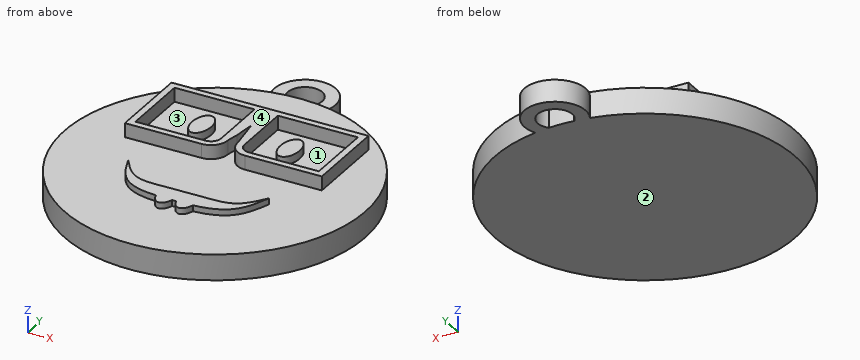
```python
from build123d import *

# Parameters (mm, degrees)
F0_R     = 75.0928281094
F2_DEPTH = 12.9
F3_DEPTH = 15.9
F5_DEPTH = 4
F6_R     = 15.2965579627
F6_R_2   = 8.6311016996
F7_DEPTH = 11
F9_DEPTH = 7


with BuildPart() as f2:
    # F0 (on Top) → F2 (new body)
    with BuildSketch(Plane.XY):
        Circle(F0_R)
    extrude(amount=F2_DEPTH)

    # F1 (on face) → F3 (join)
    with BuildSketch(Plane.XY):
        with BuildLine():
            add(Edge.make_bspline(
                [(-35.2451838553, -14.5340962335), (-32.0518207836, -19.1964482892), (-26.2372639575, -27.9738789108), (-14.7014562583, -27.6842216687), (-9.08471609, -27.5584450171)],
                knots=[0, 0, 0, 0, 0.4527149803, 0.8127890997, 0.8127890997, 0.8127890997, 0.8127890997], degree=3))
            add(Edge.make_bspline(
                [(-35.2451838553, -14.5340962335), (-32.8115077506, -21.3914317712), (-28.4404924532, -32.6892135381), (-15.405757475, -35.9303240461), (-9.2133200428, -36.2957460358)],
                knots=[0, 0, 0, 0, 0.4690101989, 0.827322276, 0.827322276, 0.827322276, 0.827322276], degree=3))
            add(Edge.make_bspline(
                [(-9.08471609, -27.5584450171), (-10.3725503531, -31.8579406773), (-9.2133200428, -36.2957460358)],
                knots=[1.0400212004, 1.0400212004, 1.0400212004, 2.0439012187, 2.0439012187, 2.0439012187], degree=2, weights=[1, 0.8766508211, 1]))
        make_face()
        with BuildLine():
            add(Edge.make_bspline(
                [(-9.08471609, -27.5584450171), (-10.3725503531, -31.8579406773), (-9.2133200428, -36.2957460358)],
                knots=[1.0400212004, 1.0400212004, 1.0400212004, 2.0439012187, 2.0439012187, 2.0439012187], degree=2, weights=[1, 0.8766508211, 1]))
            add(Edge.make_bspline(
                [(-9.2133200428, -36.2957460358), (-6.5297495568, -36.4541062417), (-3.7434296225, -36.417470813), (-0.9420935331, -36.2243297496)],
                knots=[0.827322276, 0.827322276, 0.827322276, 0.827322276, 0.9826013119, 0.9826013119, 0.9826013119, 0.9826013119], degree=3))
            add(Edge.make_bspline(
                [(-0.9420935331, -36.2243297496), (0.1851268686, -31.8136655998), (-1.0889131788, -27.559237201)],
                knots=[4.2480963919, 4.2480963919, 4.2480963919, 5.2430629887, 5.2430629887, 5.2430629887], degree=2, weights=[1, 0.8787863524, 1]))
            add(Edge.make_bspline(
                [(-9.08471609, -27.5584450171), (-6.5062543312, -27.5007050689), (-3.8211027643, -27.4435013669), (-1.0889131788, -27.559237201)],
                knots=[0.8127890997, 0.8127890997, 0.8127890997, 0.8127890997, 0.9780873545, 0.9780873545, 0.9780873545, 0.9780873545], degree=3))
        make_face()
        with BuildLine():
            add(Edge.make_bspline(
                [(-9.2133200428, -36.2957460358), (-6.5297495568, -36.4541062417), (-3.7434296225, -36.417470813), (-0.9420935331, -36.2243297496)],
                knots=[0.827322276, 0.827322276, 0.827322276, 0.827322276, 0.9826013119, 0.9826013119, 0.9826013119, 0.9826013119], degree=3))
            add(Edge.make_bspline(
                [(-9.2133200428, -36.2957460358), (-5.2569763, -51.441557274), (-1.035979555, -36.5726214568)],
                knots=[2.0439012187, 2.0439012187, 2.0439012187, 4.204730432, 4.204730432, 4.204730432], degree=2, weights=[1, 0.4709626581, 1]))
            add(Edge.make_bspline(
                [(-1.035979555, -36.5726214568), (-0.9871093073, -36.4004705121), (-0.9420935331, -36.2243297496)],
                knots=[4.204730432, 4.204730432, 4.204730432, 4.2480963919, 4.2480963919, 4.2480963919], degree=2, weights=[1, 0.9997649334, 1]))
        make_face()
        with BuildLine():
            add(Edge.make_bspline(
                [(-0.9420935331, -36.2243297496), (0.1851268686, -31.8136655998), (-1.0889131788, -27.559237201)],
                knots=[4.2480963919, 4.2480963919, 4.2480963919, 5.2430629887, 5.2430629887, 5.2430629887], degree=2, weights=[1, 0.8787863524, 1]))
            add(Edge.make_bspline(
                [(-0.9420935331, -36.2243297496), (-0.6282097401, -36.2026887014), (-0.3141374234, -36.1790827672), (0, -36.1535660923)],
                knots=[0.9826013119, 0.9826013119, 0.9826013119, 0.9826013119, 1, 1, 1, 1], degree=3))
            add(Edge.make_bspline(
                [(0.9420935331, -36.2243297496), (0.6282097401, -36.2026887014), (0.3141374234, -36.1790827672), (0, -36.1535660923)],
                knots=[0.9826013119, 0.9826013119, 0.9826013119, 0.9826013119, 1, 1, 1, 1], degree=3))
            add(Edge.make_bspline(
                [(1.0889131788, -27.559237201), (-0.1851268686, -31.8136655998), (0.9420935331, -36.2243297496)],
                knots=[1.0401223185, 1.0401223185, 1.0401223185, 2.0350889153, 2.0350889153, 2.0350889153], degree=2, weights=[1, 0.8787863524, 1]))
            add(Edge.make_bspline(
                [(1.0889131788, -27.559237201), (0.7267224105, -27.5745796394), (0.3637050295, -27.5929611946), (0, -27.6147834957)],
                knots=[0.9780873545, 0.9780873545, 0.9780873545, 0.9780873545, 1, 1, 1, 1], degree=3))
            add(Edge.make_bspline(
                [(-1.0889131788, -27.559237201), (-0.7267224105, -27.5745796394), (-0.3637050295, -27.5929611946), (0, -27.6147834957)],
                knots=[0.9780873545, 0.9780873545, 0.9780873545, 0.9780873545, 1, 1, 1, 1], degree=3))
        make_face()
        with BuildLine():
            add(Edge.make_bspline(
                [(-0.9420935331, -36.2243297496), (-0.6282097401, -36.2026887014), (-0.3141374234, -36.1790827672), (0, -36.1535660923)],
                knots=[0.9826013119, 0.9826013119, 0.9826013119, 0.9826013119, 1, 1, 1, 1], degree=3))
            add(Edge.make_bspline(
                [(-1.035979555, -36.5726214568), (-0.9871093073, -36.4004705121), (-0.9420935331, -36.2243297496)],
                knots=[4.204730432, 4.204730432, 4.204730432, 4.2480963919, 4.2480963919, 4.2480963919], degree=2, weights=[1, 0.9997649334, 1]))
            Line((-1.035979555, -36.5726214568), (1.0563025697, -36.6434637429))
            add(Edge.make_bspline(
                [(0.9420935331, -36.2243297496), (0.9964001473, -36.4368243386), (1.0563025697, -36.6434637429)],
                knots=[2.0350889153, 2.0350889153, 2.0350889153, 2.087401476, 2.087401476, 2.087401476], degree=2, weights=[1, 0.999657944, 1]))
            add(Edge.make_bspline(
                [(0.9420935331, -36.2243297496), (0.6282097401, -36.2026887014), (0.3141374234, -36.1790827672), (0, -36.1535660923)],
                knots=[0.9826013119, 0.9826013119, 0.9826013119, 0.9826013119, 1, 1, 1, 1], degree=3))
        make_face()
        with BuildLine():
            add(Edge.make_bspline(
                [(0.9420935331, -36.2243297496), (0.9964001473, -36.4368243386), (1.0563025697, -36.6434637429)],
                knots=[2.0350889153, 2.0350889153, 2.0350889153, 2.087401476, 2.087401476, 2.087401476], degree=2, weights=[1, 0.999657944, 1]))
            add(Edge.make_bspline(
                [(1.0563025697, -36.6434637429), (4.92956003, -50.0046531742), (9.036057917, -36.9136491564)],
                knots=[2.087401476, 2.087401476, 2.087401476, 4.1612301746, 4.1612301746, 4.1612301746], degree=2, weights=[1, 0.5088789213, 1]))
            add(Edge.make_bspline(
                [(9.036057917, -36.9136491564), (9.1308451493, -36.6114792608), (9.2133200428, -36.2957460358)],
                knots=[4.1612301746, 4.1612301746, 4.1612301746, 4.2392840885, 4.2392840885, 4.2392840885], degree=2, weights=[1, 0.999238545, 1]))
            add(Edge.make_bspline(
                [(9.2133200428, -36.2957460358), (6.5297495568, -36.4541062417), (3.7434296225, -36.417470813), (0.9420935331, -36.2243297496)],
                knots=[0.827322276, 0.827322276, 0.827322276, 0.827322276, 0.9826013119, 0.9826013119, 0.9826013119, 0.9826013119], degree=3))
        make_face()
        with BuildLine():
            add(Edge.make_bspline(
                [(1.0889131788, -27.559237201), (-0.1851268686, -31.8136655998), (0.9420935331, -36.2243297496)],
                knots=[1.0401223185, 1.0401223185, 1.0401223185, 2.0350889153, 2.0350889153, 2.0350889153], degree=2, weights=[1, 0.8787863524, 1]))
            add(Edge.make_bspline(
                [(9.2133200428, -36.2957460358), (6.5297495568, -36.4541062417), (3.7434296225, -36.417470813), (0.9420935331, -36.2243297496)],
                knots=[0.827322276, 0.827322276, 0.827322276, 0.827322276, 0.9826013119, 0.9826013119, 0.9826013119, 0.9826013119], degree=3))
            add(Edge.make_bspline(
                [(9.2133200428, -36.2957460358), (10.3725503531, -31.8579406773), (9.08471609, -27.5584450171)],
                knots=[4.2392840885, 4.2392840885, 4.2392840885, 5.2431641067, 5.2431641067, 5.2431641067], degree=2, weights=[1, 0.8766508211, 1]))
            add(Edge.make_bspline(
                [(9.08471609, -27.5584450171), (6.5062543312, -27.5007050689), (3.8211027643, -27.4435013669), (1.0889131788, -27.559237201)],
                knots=[0.8127890997, 0.8127890997, 0.8127890997, 0.8127890997, 0.9780873545, 0.9780873545, 0.9780873545, 0.9780873545], degree=3))
        make_face()
        with BuildLine():
            add(Edge.make_bspline(
                [(9.2133200428, -36.2957460358), (10.3725503531, -31.8579406773), (9.08471609, -27.5584450171)],
                knots=[4.2392840885, 4.2392840885, 4.2392840885, 5.2431641067, 5.2431641067, 5.2431641067], degree=2, weights=[1, 0.8766508211, 1]))
            add(Edge.make_bspline(
                [(35.2451838553, -14.5340962335), (32.8115077506, -21.3914317712), (28.4404924532, -32.6892135381), (15.405757475, -35.9303240461), (9.2133200428, -36.2957460358)],
                knots=[0, 0, 0, 0, 0.4690101989, 0.827322276, 0.827322276, 0.827322276, 0.827322276], degree=3))
            add(Edge.make_bspline(
                [(35.2451838553, -14.5340962335), (32.0518207836, -19.1964482892), (26.2372639575, -27.9738789108), (14.7014562583, -27.6842216687), (9.08471609, -27.5584450171)],
                knots=[0, 0, 0, 0, 0.4527149803, 0.8127890997, 0.8127890997, 0.8127890997, 0.8127890997], degree=3))
        make_face()
    extrude(amount=F3_DEPTH)

    # F4 (on face) → F5 (join)
    with BuildSketch(Plane.XY.offset(12.9)):
        with BuildLine():
            add(Edge.make_bspline(
                [(-22.082677111, 36.2915284932), (-30.3896638277, 36.2915284932), (-26.2361704694, 23.4395088628), (-22.082677111, 10.5874892324), (-17.9291837527, 23.4395088628), (-13.7756903943, 36.2915284932), (-22.082677111, 36.2915284932)],
                knots=[0, 0, 0, 2.0943951024, 2.0943951024, 4.1887902048, 4.1887902048, 6.2831853072, 6.2831853072, 6.2831853072], degree=2, weights=[1, 0.5, 1, 0.5, 1, 0.5, 1]))
        make_face()
        with BuildLine():
            add(Edge.make_bspline(
                [(22.082677111, 36.2915284932), (13.7756903943, 36.2915284932), (17.9291837527, 23.4395088628), (22.082677111, 10.5874892324), (26.2361704694, 23.4395088628), (30.3896638277, 36.2915284932), (22.082677111, 36.2915284932)],
                knots=[0, 0, 0, 2.0943951024, 2.0943951024, 4.1887902048, 4.1887902048, 6.2831853072, 6.2831853072, 6.2831853072], degree=2, weights=[1, 0.5, 1, 0.5, 1, 0.5, 1]))
        make_face()
    extrude(amount=F5_DEPTH)

    # F6 (on Top) → F7 (join)
    with BuildSketch(Plane.XY):
        with Locations((0, 80.6815698743)):
            Circle(F6_R)
        with Locations((0, 80.6815698743)):
            Circle(F6_R_2, mode=Mode.SUBTRACT)
    extrude(amount=F7_DEPTH)

    # F8 (on face) → F9 (join)
    with BuildSketch(Plane.XY.offset(12.9)):
        with BuildLine():
            Line((-2.4189469405, 49.3257313765), (-49.2189481235, 49.3257313765))
            Line((-49.2189481235, 49.3257313765), (-49.2189481235, 7.5257301935))
            Line((-49.2189481235, 7.5257301935), (-10.818947532, 7.5257301935))
            ThreePointArc((-10.818947532, 7.5257301935), (-4.8792501517, 9.9860334048), (-2.4189469405, 15.925730785))
            Line((-2.4189469405, 15.925730785), (-1.2094734702, 22.000117611))
            Line((-1.2094734702, 22.000117611), (0, 32.6257310808))
            Line((0, 32.6257310808), (2.4189469405, 15.925730785))
            ThreePointArc((2.4189469405, 15.925730785), (4.8792501517, 9.9860334048), (10.818947532, 7.5257301935))
            Line((10.818947532, 7.5257301935), (49.2189481235, 7.5257301935))
            Line((49.2189481235, 7.5257301935), (49.2189481235, 49.3257313765))
            Line((49.2189481235, 49.3257313765), (2.4189469405, 49.3257313765))
            Line((2.4189469405, 49.3257313765), (-2.4189469405, 49.3257313765))
        make_face()
        with BuildLine():
            Line((-45.818947532, 10.925730785), (-45.818947532, 45.925730785))
            Line((-45.818947532, 45.925730785), (-5.818947532, 45.925730785))
            Line((-5.818947532, 45.925730785), (-5.818947532, 15.925730785))
            ThreePointArc((-5.818947532, 15.925730785), (-7.2834136261, 12.3901968791), (-10.818947532, 10.925730785))
            Line((-10.818947532, 10.925730785), (-45.818947532, 10.925730785))
        make_face(mode=Mode.SUBTRACT)
        with BuildLine():
            Line((5.818947532, 15.925730785), (5.818947532, 45.925730785))
            Line((5.818947532, 45.925730785), (45.818947532, 45.925730785))
            Line((45.818947532, 45.925730785), (45.818947532, 10.925730785))
            Line((45.818947532, 10.925730785), (10.818947532, 10.925730785))
            ThreePointArc((10.818947532, 10.925730785), (7.2834136261, 12.3901968791), (5.818947532, 15.925730785))
        make_face(mode=Mode.SUBTRACT)
    extrude(amount=F9_DEPTH)


solid = f2.part
```
Build history of the part. All positions in model axes, mm. Face numbers are marked on the shaded views. A direction names the side the tool comes from. Coordinates: 2 decimals unless noted, no trailing zeros. Order: outer loops, then holes, each group sorted by start corner. A loop starts at its lowest first (then second) coordinate and runs counter-clockwise, first axis right, second up.
Item 1: Saw through at C-C on z = 7.25. List the corners of the cut face in (x, y).
Filled in:
outline: (-13.68, 73.84) arc R75.09 ccw (long way) to (13.68, 73.84) arc R15.3 ccw (long way) to start; hole (-6.34, 74.82) arc R75.09 cw to (6.34, 74.82) arc R8.63 ccw (long way) to start
Item 2: Mould opens along Y. For the marked faces 3 and 4 say: released by +Y, released by -Y, zero draft, split by the parting line, or undercut.
Filled in:
face 3: undercut
face 4: zero draft
Item 3: Saw through at B-B on y = 0. List the corners of the cut face in (x, z), then the cut area to 3 significant figures.
Filled in:
outline: (-75.09, 0) - (75.09, 0) - (75.09, 12.9) - (-75.09, 12.9) - close
area: 1,940 mm2
Item 4: Saw through at D-D on x = 62.5. List the corners of the cut face in (y, z).
Filled in:
outline: (-41.63, 0) - (41.63, 0) - (41.63, 12.9) - (-41.63, 12.9) - close
Item 5: Drill centre lines: L1, parallel to Y at x = 0, z = 2.75; L2, parallel to X at y = 33, z = 15.25; L3, parallel to Y at x = 43, z = 13.25. Where is each one in solid material? Low to high.
Filled in:
L1: y = -75.09 to 75.09, 89.31 to 95.98
L2: x = -49.22 to -45.82, -25.86 to -18.3, -5.82 to 5.82, 18.3 to 25.86, 45.82 to 49.22
L3: y = 7.53 to 10.93, 45.93 to 49.33
Item 6: Tool access for the marked faces 1 and 2: list every direction of +Z, -Z, +X, -X, +Y, -Y with a clear straight run to the whole face (end or side of a thin tool).
Filled in:
face 1: +Z
face 2: -Z, +X, -X, +Y, -Y
Item 7: Drop flat-ended pins along their axis: pin 1 Ø3.5 at (y, z) = (35, 15) entering from -X; pin 2 Ø4 at (y, z) = (-9.5, 8) entering from +X; pin 3 Ø7.5 at (y, z) = (27, 15) entering from -X; pin 4 Ø10.5 at (x, y) = (0, 80.68) entering from +Z. Give the stop position or say it passes through.
Filled in:
pin 1: stops at x = -49.22
pin 2: stops at x = 74.72
pin 3: stops at x = -71.19
pin 4: passes through
Item 8: Saw through at A-A on y = 79.5. List the corners of the cut face in (x, z), then the cut area to 3 significant figures.
Filled in:
outline: (-15.25, 0) - (-8.55, 0) - (-8.55, 11) - (-15.25, 11) - close; (8.55, 0) - (15.25, 0) - (15.25, 11) - (8.55, 11) - close
area: 147 mm2
